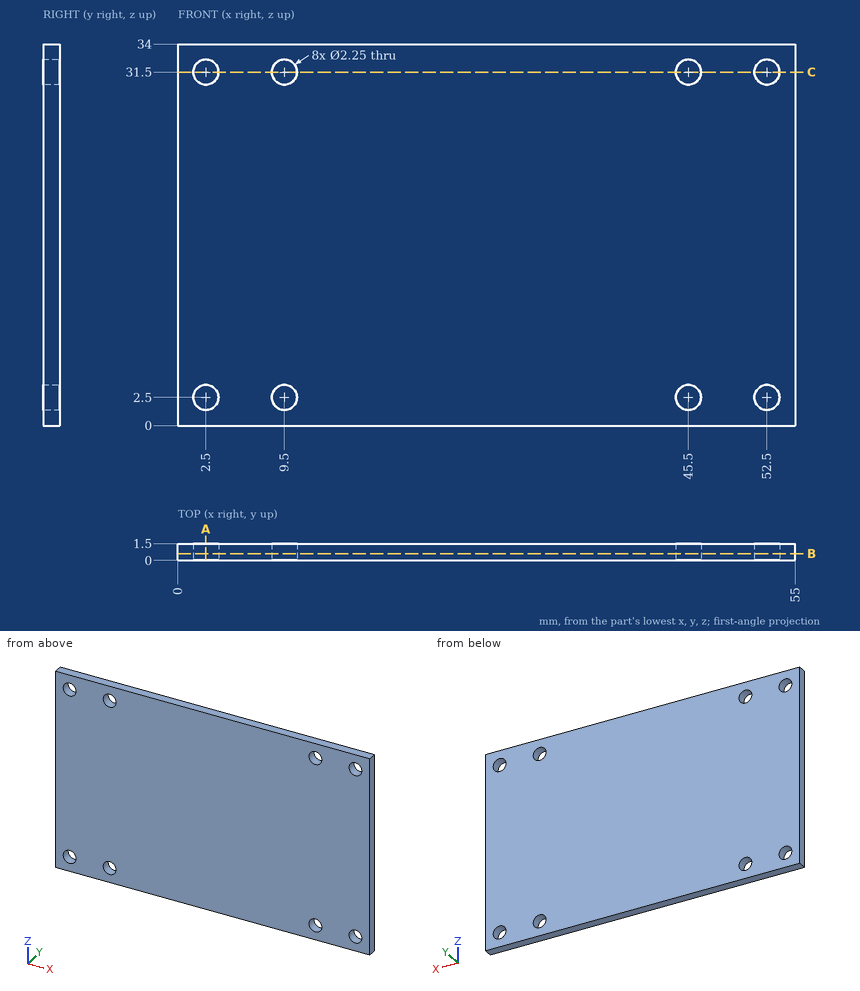
Design review of the part shown in the three views and the two pictorial views. Dimensions are in mm from the part's minimum x, y and z. Give positions to 0.01 mm unless a question says otherwise; leave off trailing zeros. Loops run counter-clockwise (first coordinate to the right, second up) from the corner with the lowest first, then second, coordinate; pieces in that order, holes last. Notation, with made-up numbers: M 64,4.5 L 120,4.5 A20 cw 120,41.5 Z; hole C 59,88 d11. An arc over 180 degrees is marked long. Write item = value, one per line.
Q1. We need section C-C (z = 31.5). Give the boundary of the cut face in (x, y) (3 decimals).
Output values:
outline = M 0,0 L 1.375,0 L 1.375,1.5 L 0,1.5 Z; M 3.625,0 L 8.375,0 L 8.375,1.5 L 3.625,1.5 Z; M 10.625,0 L 44.375,0 L 44.375,1.5 L 10.625,1.5 Z; M 46.625,0 L 51.375,0 L 51.375,1.5 L 46.625,1.5 Z; M 53.625,0 L 55,0 L 55,1.5 L 53.625,1.5 Z
Q2. Insertion check: pin 1 (1.3 mm diameter, centred on x = 2.5, z = 31.5, fed in from -Y). The pin has a flat end and moves straight along its axis. Give the tip position at first contact, or say it passes through.
Output values:
pin_1 = through
Q3. We need section B-B (y = 0.6). Count the separate pieces of the cut face and the enclosed holes in it, plus the area to 3 significant figures.
Output values:
separate_pieces = 1
enclosed_holes = 8
area = 1,840 mm^2
Q4. We need section A-A (x = 2.5). Give the boundary of the cut face in (y, z) (3 decimals), plus the area to 4 significant figures.
Output values:
outline = M 0,0 L 1.5,0 L 1.5,1.375 L 0,1.375 Z; M 0,3.625 L 1.5,3.625 L 1.5,30.375 L 0,30.375 Z; M 0,32.625 L 1.5,32.625 L 1.5,34 L 0,34 Z
area = 44.25 mm^2
Q5. To check wall thickness, follow line 1 (X direction, y = 0.35, z = 31.5) (3 decimals); line 2 (Z direction, x = 9.5, y = 0.55) (3 decimals); line 3 (X direction, y = 1.2, z = 2). State the ranges of each line that lie inside material, in increasing order. Write a range as [from, to].
Output values:
line_1 = [0, 1.375], [3.625, 8.375], [10.625, 44.375], [46.625, 51.375], [53.625, 55]
line_2 = [0, 1.375], [3.625, 30.375], [32.625, 34]
line_3 = [0, 1.49], [3.51, 8.49], [10.51, 44.49], [46.51, 51.49], [53.51, 55]
